The listing builds one solid part. Answer for the finished solid, in the listing's coordinates (mm). A direction names the side the tool comes from. Round coordinates to 2 decimals unless told otherwise and drop trailing zeros. Loops run counter-clockwise (first coordinate to the right, second up) from the corner with the lowest first, then second, coordinate; pieces in that order, holes last. Notation, with made-up numbers: M 46.5,56 L 62.5,56 A9 ccw 62.5,62 Z; hole C 39,60.25 d4. An arc over 180 degrees is marked long. Answer as a JSON object with one key per item and string values.
```python
from build123d import *

# Parameters (mm, degrees)
F2_DEPTH = 11.2
F3_R     = 8
F4_DEPTH = 80


with BuildPart() as f2:
    # F1 (on Top) → F2 (new body)
    with BuildSketch(Plane.XY):
        Polygon((7.3900834456, 12.8), (-7.3900834456, 12.8), (-14.7801668913, 0), (-7.3900834456, -12.8), (7.3900834456, -12.8), (14.7801668913, 0), align=None)
    extrude(amount=F2_DEPTH)

    # F3 (on Top) → F4 (join)
    with BuildSketch(Plane.XY):
        Circle(F3_R)
    extrude(amount=-F4_DEPTH)

    # F5 (on Right) → F6 (revolve, cut)
    with BuildSketch(Plane.YZ):
        with BuildLine():
            Line((30, 0), (30, 20))
            Line((30, 20), (0, 20))
            Line((0, 20), (0, 15.8325018302))
            ThreePointArc((0, 15.8325018302), (12.5827269819, 11.3784010225), (19.5609805226, 0))
            Line((19.5609805226, 0), (30, 0))
        make_face()
    revolve(axis=Axis((0, 0, 17.9162509151), (0, 0, -1)), mode=Mode.SUBTRACT)


solid = f2.part
```
Item 1: Which of the six approach directions +Z, -Z, +X, -X, +Y, -Y give full straight-line access (tool end or side, diameter ignored) to faces 1 (the face through (-1.73, -7.81, -39.44)), 2 (the face through (0, 0, -80))?
Values follow:
{"face 1": "-Z", "face 2": "-Z, +X, -X, +Y, -Y"}
Item 2: The part is cut by section A-A (y = -2.5). Give the vertices of the cut face in (x, z).
Values follow:
{"outline": "M -13.34,0 L -7.6,0 L -7.6,-80 L 7.6,-80 L 7.6,0 L 13.34,0 L 13.34,10.53 A19.84 ccw 12.55,11.2 L -12.55,11.2 A19.84 ccw -13.34,10.53 Z"}
Item 3: Straight lines are drawn through the part: line 1 (Z direction, x = 7.25, y = 8.5); line 2 (Y direction, x = 0.5, z = -43.5); line 3 (X direction, y = 7.5, z = 6). For each, find the intervals that lie inside material, in ascending order.
Values follow:
{"line 1": "0 to 11.2", "line 2": "-7.98 to 7.98", "line 3": "-10.45 to 10.45"}
Item 4: The part is cut by section B-B (z = -52.5). Give the vertices of the cut face in (x, y), then the cut area to 3 significant figures.
Values follow:
{"outline": "C 0,0 d16", "area": "201 mm^2"}
Item 5: Flat-ended cylindrical pins translate along their axes: P1, Ø2, axis at y = 2.5, z = -3, coming from the -X side; P2, Ø8, axis at x = -2, z = -52.5, coming from the -Y side; P3, Ø10, axis at x = 11, y = -10, coming from the -Z side. Find the tip coordinate at first contact, or state that the pin passes through.
Values follow:
{"P1": "x = -7.86", "P2": "y = -8", "P3": "z = 0"}
